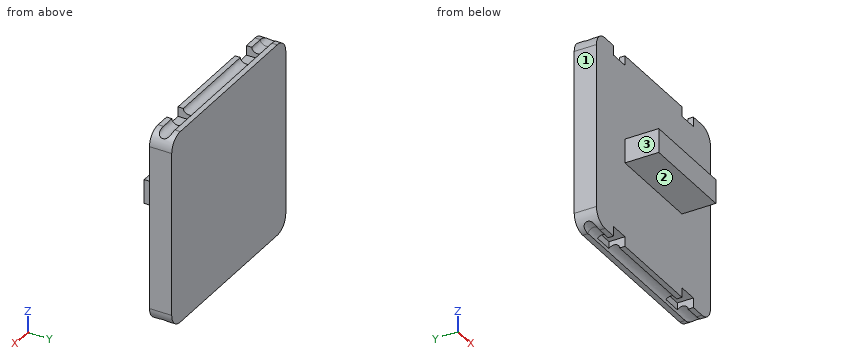
Autodesk Inventor part; units mm, degrees
ref_plane "Arbeitsebene1" through (-17, 4, 20) normal (1, 0, 0) x (0, -1, 0)
ref_plane "YZ Plane" through (0, 0, 0) normal (1, 0, 0) x (0, 1, 0)
ref_plane "XZ Plane" through (0, 0, 0) normal (0, 1, 0) x (-1, 0, 0)
sketch "Sketch1" plane through (0, 0, 0) normal (0, 1, 0) x (-1, 0, 0)
  line L0 (20, 20) -> (-20, 20)
  line L1 (-20, 20) -> (-20, -20)
  line L2 (-20, -20) -> (20, -20)
  line L3 (20, -20) -> (20, 20)
  circle A0 centre (12.5, 12.5) radius 4.25
  circle A1 centre (12.5, -12.5) radius 4.25
  circle A2 centre (-12.5, -12.5) radius 4.25
  circle A3 centre (-12.5, 12.5) radius 4.25
  line L4 (20, 0) -> (-20, 0) construction
  line L5 (0, 20) -> (0, -20) construction
  point P0 (0, 0)
  dimension "d0" = 40
  dimension "d1" = 40
  dimension "d2" = 8.5
  dimension "d3" = 25
  dimension "d4" = 25
extrude "Extrusion2" add sketch "Sketch1" along normal blind 2 contours L3 L2 L1 L0 | A0 | A1 | A2 | A3
sketch "Sketch2" plane through (0, 0, 0) normal (0, -1, 0) x (1, 0, 0)
  line L0 (20, 20) -> (20, -20)
  line L1 (-20, 20) -> (20, 20)
  line L2 (-20, -20) -> (-20, 20)
  line L3 (20, -20) -> (-20, -20)
  point P0 (0, 0)
extrude "Extrusion3" add sketch "Sketch2" along normal blind 0.6
sketch "Sketch3" plane through (0, 2, 0) normal (0, 1, 0) x (1, 0, 0)
  line L0 (-20, 20) -> (-20, -20)
  line L1 (-20, -20) -> (20, -20)
  line L2 (20, -20) -> (20, 20)
  line L3 (20, 20) -> (-20, 20)
  point P0 (0, 0)
extrude "Extrusion4" add sketch "Sketch3" along normal blind 2
fillet "Fillet1" radius 3 4 edges at (-20, 1.7, 20) (-20, 1.7, -20) (20, 1.7, 20) (20, 1.7, -20)
ref_plane "Arbeitsebene1" through (-17, 4, 20) normal (1, 0, 0) x (0, -1, 0)
sketch "Skizze5" plane through (-17, 4, 20) normal (1, 0, 0) x (0, -1, 0)
  line L0 (0, 0) -> (4.6, 0) construction
  line L1 (0, 0) -> (0, 3) construction
  line L2 (0.7, 0) -> (3.5, 0) construction
  line L3 (6.1491, 20) -> (-1.642, 20) construction
  line L4 (0, 40) -> (4.6, 40) construction
  line L5 (0.7, 40) -> (3.5, 40) construction
  line L6 (2.3, 0) -> (2.3, 4.6722) construction
  ellipse E0 centre (2.3, 0) end of major axis (3.5, 0) minor radius 1
  line L7 (1.1, 0) -> (3.5, 0)
  line L8 (0, 40) -> (4.6, 40) construction
  line L9 (0.7, 40) -> (3.5, 40) construction
  ellipse E1 centre (2.3, 40) end of major axis (3.5, 40) minor radius 1
  line L10 (1.1, 40) -> (3.5, 40)
  point P0 (4, 20)
  point P1 (2.3, 1)
  dimension "d22" = 2.3
  dimension "d23" = 1.2
  dimension "d28" = 1
extrude "Extrusion7" cut sketch "Skizze5" along normal blind 37 and the other way blind 5 contours L7 E0 | E1 L10 picked at (2.3176, 0.333) picked at (2.2824, 39.667)
sketch "Skizze6" plane through (0, -0.6, 0) normal (0, -1, 0) x (1, 0, 0)
  line L0 (17, 20) -> (-17, 20)
  line L1 (-20, 17) -> (-20, -17) construction
  line L2 (-14, 20) -> (-14, 18)
  line L3 (-14, 20) -> (-10, 20)
  line L4 (0, 16.6905) -> (0, 25.5183)
  line L5 (7.2129, 0) -> (-7.9382, 0)
  line L6 (-17, 20) -> (17, 20)
  line L7 (14, 20) -> (10, 20)
  line L8 (17, -20) -> (-17, -20)
  line L9 (-14, 18) -> (-10, 18)
  line L10 (-10, 18) -> (-10, 20)
  line L11 (-17, -20) -> (17, -20)
  line L12 (14, 20) -> (14, 18)
  line L13 (14, 18) -> (10, 18)
  line L14 (10, 18) -> (10, 20)
  line L15 (-14, -20) -> (-14, -18)
  line L16 (-14, -18) -> (-10, -18)
  line L17 (-10, -18) -> (-10, -20)
  line L18 (10, -18) -> (10, -20)
  line L19 (14, -18) -> (10, -18)
  line L20 (14, -20) -> (14, -18)
  point P0 (0, 0)
  point P1 (-12, 20)
  dimension "d34" = 8
  dimension "d35" = 2
  dimension "d41" = 2
  dimension "d42" = 4
extrude "Extrusion8" cut sketch "Skizze6" against normal blind 3.3
sketch "Skizze7" plane through (0, -0.6, 0) normal (0, -1, 0) x (1, 0, 0)
  line L0 (-10, 2.5) -> (10, 2.5)
  line L1 (10, 2.5) -> (10, -2.5)
  line L2 (10, -2.5) -> (-10, -2.5)
  line L3 (-10, -2.5) -> (-10, 2.5)
  line L4 (-10, 2.5) -> (10, -2.5) construction
  line L5 (10, 2.5) -> (-10, -2.5) construction
  point P0 (0, 0)
  dimension "d43" = 5
  dimension "d44" = 20
extrude "Extrusion9" add sketch "Skizze7" along normal blind 7
properties part number "IMU_mount_baseplate"
Geometry check sheet. Reference: the model listing, model coordinates, mm. Face numbers are marked on the shaded views. A direction names the side the tool comes from. Give positions to 0.01 mm unless a question says otherwise; leave off trailing zeros. Write each loop counter-clockwise with the first axis right and the second up, starting at its lowest first coordinate (ties: lowest second). Pieces come first, ordered by that corner, then holes. Notation, with made-up numbers: (43.5, 50.25) - (69.5, 50.25) arc R22 cw to (69.5, 68.25) - close; hole circle Ø8 at (87.5, 52). An arc over 180 degrees is marked (long way). Put each result on its own line as item: value.
1. Go/stop test with flat-tipped pins: pin 1 (6 mm diameter, centred on x = -10, y = -5, fed in from +Z); pin 2 (0.6 mm diameter, centred on y = 1, z = 19, fed in from -X); pin 3 (0.6 mm diameter, centred on y = 1.5, z = -18.5, fed in from -X); pin 4 (6 mm diameter, centred on y = -6, z = -13.5, fed in from -X). Record where each tip stops, or that it passes through.
Ans:
pin 1: stops at z = 2.5
pin 2: stops at x = -19.47
pin 3: stops at x = -19.75
pin 4: passes through
2. Set-up check for the marked faces 1, 2 and 3: record each of +Z, -Z, +X, -X, +Y, -Y from which the full face is reachable in a straight line by a thin tool's end or side.
Ans:
face 1: +Z, -Z, -X, +Y, -Y
face 2: -Z, +X, -X, -Y
face 3: +Z, -Z, -X, -Y
3. Thickness scan on line 1 (Z direction, x = -3.5, y = -3.25); line 2 (Y direction, x = 16.5, z = 16.5); line 3 (Z direction, x = -16, y = 2). Record the ranges inside material, lowest first.
Ans:
line 1: z = -2.5 to 2.5
line 2: y = -0.6 to 4
line 3: z = -19.03 to 19.03
4. Sectioned sample at B-B, the plane y = -2.75. Enter the section's corners in (x, z).
Ans:
outline: (-10, -2.5) - (10, -2.5) - (10, 2.5) - (-10, 2.5) - close
5. Sectioned sample at A-A, the plane z = 1. Enter the section's corners in (x, y).
Ans:
outline: (-20, -0.6) - (-10, -0.6) - (-10, -7.6) - (10, -7.6) - (10, -0.6) - (20, -0.6) - (20, 4) - (-20, 4) - close
6. Sectioned sample at C-C, the plane z = -11.5. Enter the section's corners in (x, y), plus the area to 3 significant figures.
Ans:
outline: (-20, -0.6) - (20, -0.6) - (20, 4) - (-20, 4) - close
area: 184 mm²
